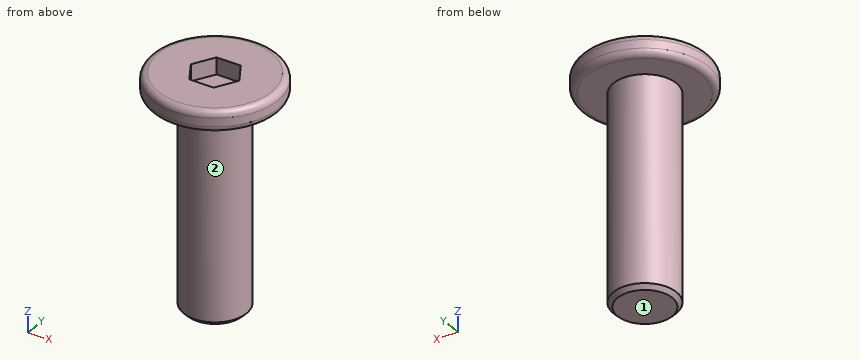
```python
from build123d import *

# Parameters (mm, degrees)
SKETCH_1_R          = 3
EXTRUDE_1_DEPTH     = 0.5
SKETCH_2_R          = 1.5
EXTRUDE_2_DEPTH     = 10
CHAMFER_1_SIZE      = 0.2
CUT_EXTRUDE_1_DEPTH = 0.8
FILLET_2_R          = 0.3


with BuildPart() as part:
    # 草图1 → 凸台-拉伸1 (new, symmetric)
    with BuildSketch(Plane.XY):
        Circle(SKETCH_1_R)
    extrude(amount=EXTRUDE_1_DEPTH, both=True)

    # 草图2 → 凸台-拉伸2 (add)
    with BuildSketch(Plane(origin=(0, 0, -0.5), x_dir=(-1, 0, 0), z_dir=(0, 0, -1))):
        Circle(SKETCH_2_R)
    extrude(amount=EXTRUDE_2_DEPTH)

    # 倒角1
    chamfer_1_edges = [part.edges().sort_by_distance(p)[0] for p in [
        (1.5, 0, -10.5),
    ]]
    chamfer(chamfer_1_edges, length=CHAMFER_1_SIZE)

    # 草图3 → 切除-拉伸1 (cut)
    with BuildSketch(Plane.XY.offset(0.5)):
        Polygon((1.154700538, 0), (0.577350269, 1), (-0.577350269, 1), (-1.154700538, 0), (-0.577350269, -1), (0.577350269, -1), align=None)
    extrude(amount=-CUT_EXTRUDE_1_DEPTH, mode=Mode.SUBTRACT)

    # 圆角2
    fillet_2_edges = [part.edges().sort_by_distance(p)[0] for p in [
        (-3, 0, -0.5),
        (-3, 0, 0.5),
    ]]
    fillet(fillet_2_edges, radius=FILLET_2_R)


solid = part.part
```
Part model, mm, in its own coordinate system. Face numbers are marked on the shaded views. A direction names the side the tool comes from. Round coordinates to 2 decimals unless told otherwise and drop trailing zeros. Write each loop counter-clockwise with the first axis right and the second up, starting at its lowest first coordinate (ties: lowest second). Pieces come first, ordered by that corner, then holes.
Item 1: Cut at B-B, the plane z = -3.5. Give the cut face in (x, y).
Results:
outline: circle Ø3 at (0, 0)
Item 2: Cut at A-A, the plane x = 0. Give the cut face in (y, z).
Results:
outline: (-3, -0.2) arc R0.3 ccw to (-2.7, -0.5) - (-1.5, -0.5) - (-1.5, -10.3) - (-1.3, -10.5) - (1.3, -10.5) - (1.5, -10.3) - (1.5, -0.5) - (2.7, -0.5) arc R0.3 ccw to (3, -0.2) - (3, 0.2) arc R0.3 ccw to (2.7, 0.5) - (1, 0.5) - (1, -0.3) - (-1, -0.3) - (-1, 0.5) - (-2.7, 0.5) arc R0.3 ccw to (-3, 0.2) - close
Item 3: Probe L1, parallel to Z at x = 1.25, y = 1.25; L2, parallel to Z at x = -0.5, y = 0.5; L3, parallel to Y at x = 1, z = -7.5. List the from-to ranges inside material, lowest first.
Results:
L1: z = -0.5 to 0.5
L2: z = -10.5 to -0.3
L3: y = -1.12 to 1.12
Item 4: Drop flat-ended pins along their axis: pin 1 Ø3 at (x, z) = (2, -4) entering from +Y; pin 2 Ø1.6 at (x, y) = (0, 0.5) entering from +Z; pin 3 Ø1.5 at (y, z) = (-2, -4.5) entering from +X; pin 4 Ø2 at (y, z) = (1, -2) entering from +X. Give the stop position or say it passes through.
Results:
pin 1: stops at y = 1.41
pin 2: stops at z = 0.5
pin 3: stops at x = 0.83
pin 4: stops at x = 1.5
Item 5: Which spindle directions (+Z, -Z, +X, -X, +Y, -Y) get a long thin tool onto all of the face, cutting with end or side? Do the marked faces 1 and 2. Say none if no direction does.
Results:
face 1: -Z, +X, -X, +Y, -Y
face 2: -Z
